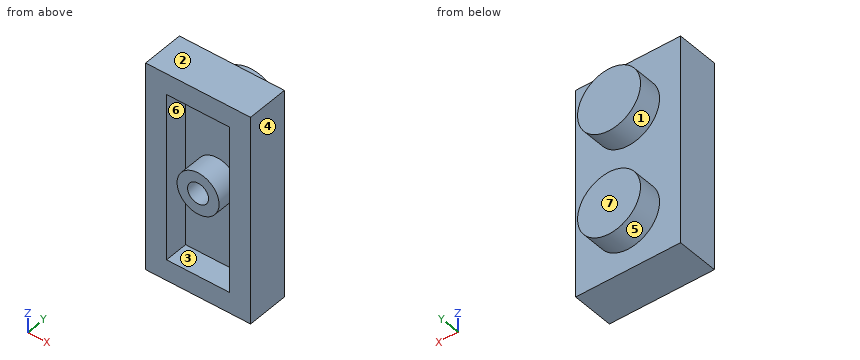
```python
from build123d import *

# Parameters (mm, degrees)
SKETCH1_W           = 8
SKETCH1_H           = 3.2
BOSS_EXTRUDE1_DEPTH = 16
SKETCH2_W           = 4.8
SKETCH2_H           = 12.8
CUT_EXTRUDE1_DEPTH  = 1.8
SKETCH3_R           = 2.4
BOSS_EXTRUDE2_DEPTH = 1.8
SKETCH4_R           = 1.6
BOSS_EXTRUDE3_DEPTH = 1.8
SKETCH5_R           = 0.8
CUT_EXTRUDE2_DEPTH  = 1.8


with BuildPart() as part:
    # Sketch1 → Boss-Extrude1 (new body)
    with BuildSketch(Plane.XY):
        with Locations((4, 1.6)):
            Rectangle(SKETCH1_W, SKETCH1_H)
    extrude(amount=BOSS_EXTRUDE1_DEPTH)

    # Sketch2 → Cut-Extrude1 (cut)
    with BuildSketch(Plane.XZ):
        with Locations((4, 8)):
            Rectangle(SKETCH2_W, SKETCH2_H)
    extrude(amount=-CUT_EXTRUDE1_DEPTH, mode=Mode.SUBTRACT)

    # Sketch3 → Boss-Extrude2 (add)
    with BuildSketch(Plane(origin=(0, 3.2, 0), x_dir=(1, 0, 0), z_dir=(0, 1, 0))):
        with Locations(Location((4, -4, 0), (0, 0, 90))):
            Circle(SKETCH3_R)
        with Locations(Location((4, -12, 0), (0, 0, 90))):
            Circle(SKETCH3_R)
    extrude(amount=BOSS_EXTRUDE2_DEPTH)

    # Sketch4 → Boss-Extrude3 (add)
    with BuildSketch(Plane.XZ.offset(-1.8)):
        with Locations(Location((4, 8, 0), (0, 0, 270))):
            Circle(SKETCH4_R)
    extrude(amount=BOSS_EXTRUDE3_DEPTH)

    # Sketch5 → Cut-Extrude2 (cut)
    with BuildSketch(Plane.XZ):
        with Locations(Location((4, 8, 0), (0, 0, 270))):
            Circle(SKETCH5_R)
    extrude(amount=-CUT_EXTRUDE2_DEPTH, mode=Mode.SUBTRACT)


solid = part.part
```
The model under review builds one solid part; all positions refer to its coordinate system, in mm. Face numbers are marked on the shaded views. A direction names the side the tool comes from. Round coordinates to 2 decimals unless told otherwise and drop trailing zeros. Loops run counter-clockwise (first coordinate to the right, second up) from the corner with the lowest first, then second, coordinate; pieces in that order, holes last. Notation, with made-up numbers: M 45,4.25 L 51,4.25 A28 cw 51,34.25 Z; hole C -5,60 d3. An arc over 180 degrees is marked long. Write item = value, one per line.
Item 1: The part is to be moulded in two halves that separate along X. For the marked faces 1, 2, 3 and 4, say which applies: released by +X, released by -X, zero draft, split by the parting line, or undercut.
Return value:
face_1 = split by the parting line
face_2 = zero draft
face_3 = undercut
face_4 = released by +X
Item 2: Take a section at C-C on z = 4. Write out the cut boundary in (x, y), then the cut area to 3 significant figures.
Return value:
outline = M 0,0 L 1.6,0 L 1.6,1.8 L 6.4,1.8 L 6.4,0 L 8,0 L 8,3.2 L 6.4,3.2 L 6.4,5 L 1.6,5 L 1.6,3.2 L 0,3.2 Z
area = 25.6 mm2
Item 3: Insertion check: P1, Ø4, axis at x = 3, z = 8, coming from the -Y side; P2, Ø1.4, axis at x = 4, z = 8, coming from the +Y side; P3, Ø1.5, axis at y = 4, z = 5.5, coming from the +X side. Each pin has a flat end and moves straight along its axis. Give the tip position at first contact, or say it passes through.
Return value:
P1 = 0
P2 = 3.2
P3 = 6.28
Item 4: For line 1 (X direction, y = 0.7, z = 8); line 2 (X direction, y = 1.35, z = 12.25); line 3 (Y direction, x = 1, z = 7.5), list the stretches that pass through material, from the lowest coordinate up. Write a range as [from, to].
Return value:
line_1 = [0, 1.6], [2.4, 3.2], [4.8, 5.6], [6.4, 8]
line_2 = [0, 1.6], [6.4, 8]
line_3 = [0, 3.2]
Item 5: Take a section at A-A on y = 0.9. Write out the cut boundary in (x, z).
Return value:
outline = M 0,0 L 8,0 L 8,16 L 0,16 Z; C 4,8 d3.2; hole M 1.6,1.6 L 6.4,1.6 L 6.4,14.4 L 1.6,14.4 Z; hole C 4,8 d1.6
Item 6: Take a section at D-D on y = 3.5. Write out the cut boundary in (x, z), then the cut area to 3 significant figures.
Return value:
outline = C 4,4 d4.8; C 4,12 d4.8
area = 36.2 mm2
Item 7: Machinability: for the marked faces 5, 6 and 7, which of the approach directions +Z, -Z, +X, -X, +Y, -Y give a long, thin tool a straight path to every point of the face, cutting with its end or side? Answer none if there is none.
Return value:
face_5 = +Y
face_6 = -Y
face_7 = +Z, -Z, +X, -X, +Y
Item 8: Take a section at B-B on x = 4. Write out the cut boundary in (y, z), then the cut area to 3 significant figures.
Return value:
outline = M 0,0 L 3.2,0 L 3.2,1.6 L 5,1.6 L 5,6.4 L 3.2,6.4 L 3.2,9.6 L 5,9.6 L 5,14.4 L 3.2,14.4 L 3.2,16 L 0,16 L 0,14.4 L 1.8,14.4 L 1.8,9.6 L 0,9.6 L 0,8.8 L 1.8,8.8 L 1.8,7.2 L 0,7.2 L 0,6.4 L 1.8,6.4 L 1.8,1.6 L 0,1.6 Z
area = 48.3 mm2
